from build123d import *

# Parameters (mm, degrees)
SKETCH1_W           = 77.5
SKETCH1_H           = 24.5
BOSS_EXTRUDE1_DEPTH = 1.25
FILLET1_R           = 1
CUT_EXTRUDE1_REACH  = 42.659
SKETCH2_R           = 1.5
SKETCH3_W           = 5.75
SKETCH3_H           = 10
BOSS_EXTRUDE2_DEPTH = 6
FILLET2_R           = 1
LPATTERN1_START     = 2.25
LPATTERN1_DEPTH     = 10
LPATTERN1_START_2   = -37.75
LPATTERN1_2_DEPTH   = 76.75


with BuildPart() as part:
    # Sketch1 → Boss-Extrude1 (new body)
    with BuildSketch(Plane(origin=(0, 0, 0), x_dir=(1, 0, 0), z_dir=(0, 1, 0))):
        Rectangle(SKETCH1_W, SKETCH1_H)
    extrude(amount=BOSS_EXTRUDE1_DEPTH)

    # Fillet1
    fillet1_edges = [part.edges().sort_by_distance(p)[0] for p in [
        (38.75, 0.625, 12.25),
        (-38.75, 0.625, 12.25),
        (-38.75, 0.625, -12.25),
        (38.75, 0.625, -12.25),
    ]]
    fillet(fillet1_edges, radius=FILLET1_R)

    # Sketch2 → Cut-Extrude1 (cut, up to next)
    with BuildSketch(Plane.XZ, mode=Mode.PRIVATE) as cut_extrude1_sk1:
        with Locations(Location((36.25, -1.75, 0), (0, 0, 270))):
            Circle(SKETCH2_R)
    cut_extrude1_tool1 = extrude(cut_extrude1_sk1.sketch, amount=-CUT_EXTRUDE1_REACH, mode=Mode.PRIVATE) & part.part
    # Sketch2 → Cut-Extrude1 (cut, up to next)
    with BuildSketch(Plane.XZ, mode=Mode.PRIVATE) as cut_extrude1_sk2:
        with Locations(Location((-36.25, -1.75, 0), (0, 0, 90))):
            Circle(SKETCH2_R)
    cut_extrude1_tool2 = extrude(cut_extrude1_sk2.sketch, amount=-CUT_EXTRUDE1_REACH, mode=Mode.PRIVATE) & part.part
    add(cut_extrude1_tool1.solids().sort_by_distance((36.25, 0, -1.75))[0], mode=Mode.SUBTRACT)
    add(cut_extrude1_tool2.solids().sort_by_distance((-36.25, 0, -1.75))[0], mode=Mode.SUBTRACT)

    # Sketch3 → Boss-Extrude2 (add)
    with BuildSketch(Plane.XZ):
        with Locations((-34.875, 7.25)):
            Rectangle(SKETCH3_W, SKETCH3_H)
    extrude(amount=BOSS_EXTRUDE2_DEPTH)

    # Fillet2
    fillet2_edges = [part.edges().sort_by_distance(p)[0] for p in [
        (-37.75, -6, 7.25),
        (-34.875, -6, 2.25),
        (-32, -6, 7.25),
        (-34.875, -6, 12.25),
    ]]
    fillet(fillet2_edges, radius=FILLET2_R)

    # LPattern1: read off the stored shape, not the designer's step
    # LPattern1 outline → LPattern1 (add)
    with BuildSketch(Plane.XY.offset(LPATTERN1_START)):
        with BuildLine():
            ThreePointArc((-27.75, -5), (-27.457106781, -5.707106781), (-26.75, -6))
            Line((-26.75, -6), (-23, -6))
            ThreePointArc((-23, -6), (-22.292893219, -5.707106781), (-22, -5))
            Line((-22, -5), (-22, 0))
            Line((-22, 0), (-27.75, 0))
            Line((-27.75, 0), (-27.75, -5))
        make_face()
        with BuildLine():
            Line((38, 0), (32.25, 0))
            Line((32.25, 0), (32.25, -5))
            ThreePointArc((32.25, -5), (32.542893219, -5.707106781), (33.25, -6))
            Line((33.25, -6), (37, -6))
            ThreePointArc((37, -6), (37.707106781, -5.707106781), (38, -5))
            Line((38, -5), (38, 0))
        make_face()
        with BuildLine():
            Line((28, 0), (22.25, 0))
            Line((22.25, 0), (22.25, -5))
            ThreePointArc((22.25, -5), (22.542893219, -5.707106781), (23.25, -6))
            Line((23.25, -6), (27, -6))
            ThreePointArc((27, -6), (27.707106781, -5.707106781), (28, -5))
            Line((28, -5), (28, 0))
        make_face()
        with BuildLine():
            Line((18, 0), (12.25, 0))
            Line((12.25, 0), (12.25, -5))
            ThreePointArc((12.25, -5), (12.542893219, -5.707106781), (13.25, -6))
            Line((13.25, -6), (17, -6))
            ThreePointArc((17, -6), (17.707106781, -5.707106781), (18, -5))
            Line((18, -5), (18, 0))
        make_face()
        with BuildLine():
            Line((8, 0), (2.25, 0))
            Line((2.25, 0), (2.25, -5))
            ThreePointArc((2.25, -5), (2.542893219, -5.707106781), (3.25, -6))
            Line((3.25, -6), (7, -6))
            ThreePointArc((7, -6), (7.707106781, -5.707106781), (8, -5))
            Line((8, -5), (8, 0))
        make_face()
        with BuildLine():
            Line((-2, 0), (-7.75, 0))
            Line((-7.75, 0), (-7.75, -5))
            ThreePointArc((-7.75, -5), (-7.457106781, -5.707106781), (-6.75, -6))
            Line((-6.75, -6), (-3, -6))
            ThreePointArc((-3, -6), (-2.292893219, -5.707106781), (-2, -5))
            Line((-2, -5), (-2, 0))
        make_face()
        with BuildLine():
            Line((-12, 0), (-17.75, 0))
            Line((-17.75, 0), (-17.75, -5))
            ThreePointArc((-17.75, -5), (-17.457106781, -5.707106781), (-16.75, -6))
            Line((-16.75, -6), (-13, -6))
            ThreePointArc((-13, -6), (-12.292893219, -5.707106781), (-12, -5))
            Line((-12, -5), (-12, 0))
        make_face()
    extrude(amount=LPATTERN1_DEPTH)

    # LPattern1 2 outline → LPattern1 2 (cut)
    with BuildSketch(Plane.YZ.offset(LPATTERN1_START_2)):
        with BuildLine():
            Line((-6, 2.25), (-5, 2.25))
            ThreePointArc((-5, 2.25), (-5.707106781, 2.542893219), (-6, 3.25))
            Line((-6, 3.25), (-6, 2.25))
        make_face()
        with BuildLine():
            Line((-6, 12.25), (-6, 11.25))
            ThreePointArc((-6, 11.25), (-5.707106781, 11.957106781), (-5, 12.25))
            Line((-5, 12.25), (-6, 12.25))
        make_face()
    extrude(amount=LPATTERN1_2_DEPTH, mode=Mode.SUBTRACT)


solid = part.part
Could you check a few things on this model? Use its own coordinates, in mm. A direction names the side the tool comes from. Give positions to 0.01 mm unless a question says otherwise; leave off trailing zeros. Write each loop counter-clockwise with the first axis right and the second up, starting at its lowest first coordinate (ties: lowest second). Pieces come first, ordered by that corner, then holes. Notation, with made-up numbers: (11, 59.25) -> (37, 59.25) arc R18 cw to (37, 90.25) -> close; hole circle Ø4 at (0, 83). An arc over 180 degrees is marked (long way). Answer as CSV lines item,"result". Start each with the question number.
(1) I'm going to push flat-ended pins straight in: pin 1 Ø1.5 at (y, z) = (-3.5, 4.5) entering from +X; pin 2 Ø2.5 at (y, z) = (-2.5, 7) entering from -X; pin 3 Ø1.8 at (x, z) = (-36.25, -1.75) entering from -Y; pin 4 Ø4 at (x, y) = (34, -3) entering from -Z. Where does each tip first touch, or does it pass through?
(2) Please list where these lines run through material, in increasing order: line 1 (X direction, y = 0.9, z = -1.75); line 2 (Z direction, x = -36.25, y = 0.3); line 3 (Y direction, x = 20.5, z = 10).
(3) If we section it at D-D, the plane x = 1: Write out the boundary of the cut face in (y, z), and give its area (3 significant figures).
(4) Which directions (+Z, -Z, +X, -X, +Y, -Y) give clear straight access to the entire face, cutting with the end or side of a thin tool? Please do faces 1 (the face through (-1, 0, -3)), 2 (the face through (-1, 1, -12.25)), 3 (the face through (-25, -2, 2.25)), 4 (the face through (32.25, -2, 7)).
(5) If we section it at A-A, the plane x = 36.25: Write out the boundary of the cut face in (y, z), and give its area (3 significant figures).
(6) If we mould it in two halves opening along X, with no side actions, what happens to faces 5 (the face through (38.75, 1, 0)), 6 (the face through (-27.75, -2, 7)), 7 (the face through (-25, -6, 7))? For each: +X half, -X half, draft (parallel to the pull), parting line (faces both ways), or undercut.
(7) If we section it at B-B, the plane z = -1.75: Write out the boundary of the cut face in (x, y).
(8) If we section it at C-C, the plane y = -2: Give the number of separate pieces and of enclosed holes in the cut face, and give its area (3 significant figures).
Answer list:
1,pin 1,"x = 38"
1,pin 2,"x = -37.75"
1,pin 3,"through"
1,pin 4,"z = 2.25"
2,line 1,"-38.75 to -37.75, -34.75 to 34.75, 37.75 to 38.75"
2,line 2,"-12.25 to -3.25, -0.25 to 12.25"
2,line 3,"0 to 1.25"
3,outline,"(0, -12.25) -> (1.25, -12.25) -> (1.25, 12.25) -> (0, 12.25) -> close"
3,area,"30.6 mm^2"
4,face 1,"-Z, -Y"
4,face 2,"-Z, +X, -X, +Y, -Y"
4,face 3,"-Z, +X, -X, -Y"
4,face 4,"+Z, -Z, -Y"
5,outline,"(-6, 3.25) arc R1 ccw to (-5, 2.25) -> (0, 2.25) -> (0, -0.25) -> (1.25, -0.25) -> (1.25, 12.25) -> (-5, 12.25) arc R1 ccw to (-6, 11.25) -> close; (0, -12.25) -> (1.25, -12.25) -> (1.25, -3.25) -> (0, -3.25) -> close"
5,area,"86.4 mm^2"
6,face 5,"+X half"
6,face 6,"undercut"
6,face 7,"draft"
7,outline,"(-38.75, 0) -> (-37.75, 0) -> (-37.75, 1.25) -> (-38.75, 1.25) -> close; (-34.75, 0) -> (34.75, 0) -> (34.75, 1.25) -> (-34.75, 1.25) -> close; (37.75, 0) -> (38.75, 0) -> (38.75, 1.25) -> (37.75, 1.25) -> close"
8,separate pieces,"8"
8,enclosed holes,"0"
8,area,"460 mm^2"
